The figure shows three views and two pictorial views of one solid part (mm, origin at its lowest corner). Answer the questions. Round coordinates to 2 decimals unless told otherwise and drop trailing zeros. Order: outer loops, then holes, each group sorted by start corner. A loop starts at its lowest first (then second) coordinate and runs counter-clockwise, first axis right, second up. Notation, with made-up numbers: (41.5, -3.5) -> (69.5, -3.5) arc R9 cw to (69.5, 11.5) -> close; hole circle Ø9 at (32.25, 36). An arc over 180 degrees is marked (long way). One line per item, written item: value. Start each with the question number.
1. Consider line 1 (X direction, y = 1.7, z = 81); line 2 (X direction, y = 1.05, z = 7); line 3 (Z direction, x = 76.75, y = 0.8). Determine where each line is inside the solid, lowest interval first.
2. Flat-ended cylindrical pins translate along their axes: pin 1 Ø1.5 at (x, y) = (162, 1) entering from -Z; pin 2 Ø1.5 at (x, y) = (154, 1) entering from +Z. Find the tip coordinate at first contact, or state that the pin passes through.
3. Section B-B (z = 148) is taken. Give the vertices of the cut face in (x, y), then the cut area to 4 significant figures.
4. Section A-A (y = 0.95) is taken. Give the vertices of the cut face in (x, z), then the cut area to 3 significant figures.
5. Section C-C (x = 107.5) is taken. Give the vertices of the cut face in (y, z), then the cut area to 3 significant figures.
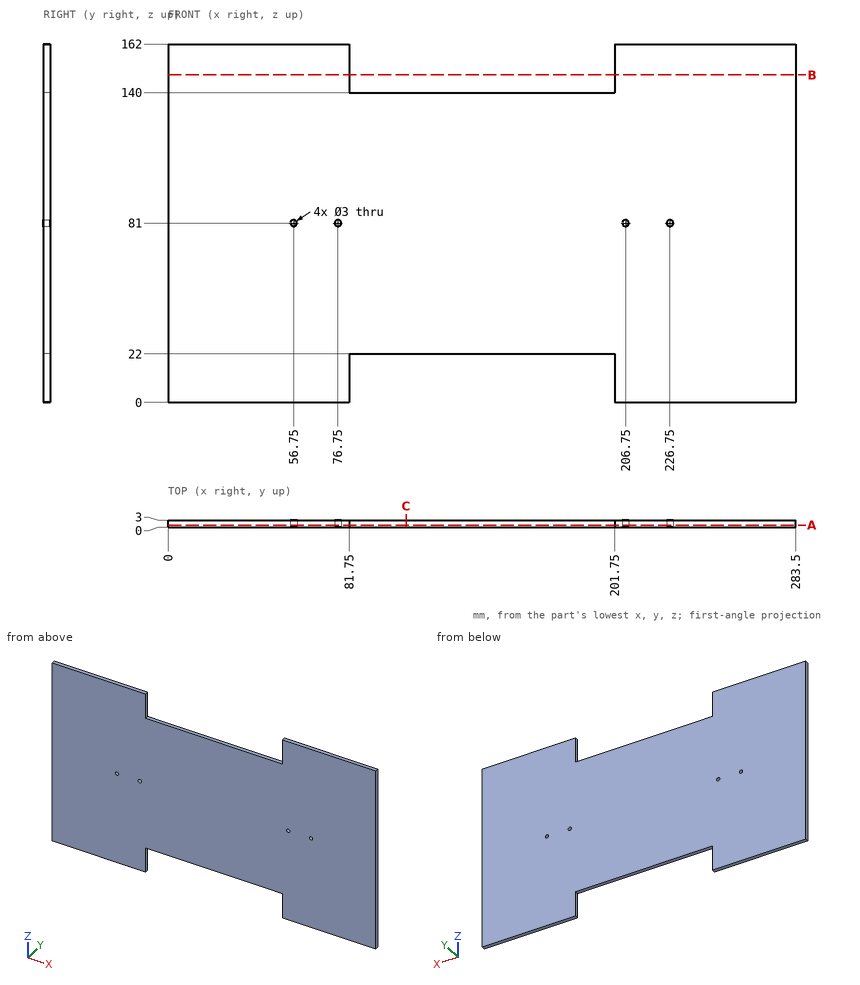
Answer:
1. line 1: 0 to 55.25, 58.25 to 75.25, 78.25 to 205.25, 208.25 to 225.25, 228.25 to 283.5
1. line 2: 0 to 81.75, 201.75 to 283.5
1. line 3: 0 to 79.5, 82.5 to 162
2. pin 1: z = 22
2. pin 2: z = 140
3. outline: (0, 0) -> (81.75, 0) -> (81.75, 3) -> (0, 3) -> close; (201.75, 0) -> (283.5, 0) -> (283.5, 3) -> (201.75, 3) -> close
3. area: 490.5 mm^2
4. outline: (0, 0) -> (81.75, 0) -> (81.75, 22) -> (201.75, 22) -> (201.75, 0) -> (283.5, 0) -> (283.5, 162) -> (201.75, 162) -> (201.75, 140) -> (81.75, 140) -> (81.75, 162) -> (0, 162) -> close; hole circle Ø3 at (56.75, 81); hole circle Ø3 at (76.75, 81); hole circle Ø3 at (206.75, 81); hole circle Ø3 at (226.75, 81)
4. area: 40,600 mm^2
5. outline: (0, 22) -> (3, 22) -> (3, 140) -> (0, 140) -> close
5. area: 354 mm^2
